Could you check a few things on this model? Use its own coordinates, in mm. A direction names the side the tool comes from. Round coordinates to 2 decimals unless told otherwise and drop trailing zeros. Loops run counter-clockwise (first coordinate to the right, second up) from the corner with the lowest first, then second, coordinate; pieces in that order, holes last.
from build123d import *

# Parameters (mm, degrees)
BOSS_EXTRUDE1_DEPTH = 300
SKETCH2_R           = 42.5
SKETCH2_W           = 5
SKETCH2_H           = 83.856690982
CUT_EXTRUDE1_DEPTH  = 349.855848061
SKETCH3_R           = 2
CUT_EXTRUDE2_DEPTH  = 349.855848061


with BuildPart() as part:
    # Sketch1 → Boss-Extrude1 (new body)
    with BuildSketch(Plane(origin=(0, 0, 0), x_dir=(0, 0, -1), z_dir=(1, 0, 0))):
        with BuildLine():
            Line((0, 0), (73.417375121, 0))
            ThreePointArc((73.417375121, 0), (79.943684732, -0.427756931), (86.358327376, -1.703708686))
            Line((86.358327376, -1.703708686), (176.592582629, -25.88190451))
            Line((176.592582629, -25.88190451), (175.816125494, -28.779681989))
            Line((175.816125494, -28.779681989), (85.58187024, -4.601486164))
            ThreePointArc((85.58187024, -4.601486164), (79.552106155, -3.402091515), (73.417375121, -3))
            Line((73.417375121, -3), (0, -3))
            Line((0, -3), (0, 0))
        make_face()
    extrude(amount=BOSS_EXTRUDE1_DEPTH)

    # Sketch2 → Cut-Extrude1 (cut, through all)
    with BuildSketch(Plane(origin=(0, 20, -5.358983849), x_dir=(1, 0, 0), z_dir=(0, 0.9659258262890681, -0.25881904510252174))):
        with Locations((48, 152.274066103)):
            Circle(SKETCH2_R)
        with Locations((252, 152.274066103)):
            Circle(SKETCH2_R)
        with Locations((48, -29.084261273)):
            Circle(SKETCH2_R)
        with Locations((252, -29.084261273)):
            Circle(SKETCH2_R)
        with Locations((2.5, 41.928345491)):
            Rectangle(SKETCH2_W, SKETCH2_H)
        with Locations((297.5, 41.928345491)):
            Rectangle(SKETCH2_W, SKETCH2_H)
    extrude(amount=-CUT_EXTRUDE1_DEPTH, mode=Mode.SUBTRACT)

    # Sketch3 → Cut-Extrude2 (cut, through all)
    with BuildSketch(Plane(origin=(0, 20, -5.358983849), x_dir=(1, 0, 0), z_dir=(0, 0.9659258262890681, -0.25881904510252174))):
        with Locations(Location((8, 87.856690982, 0), (0, 0, 270))):
            Circle(SKETCH3_R)
        with Locations(Location((8, 111.856690982, 0), (0, 0, 270))):
            Circle(SKETCH3_R)
        with Locations(Location((292, 87.856690982, 0), (0, 0, 270))):
            Circle(SKETCH3_R)
        with Locations(Location((292, 111.856690982, 0), (0, 0, 270))):
            Circle(SKETCH3_R)
    extrude(amount=-CUT_EXTRUDE2_DEPTH, mode=Mode.SUBTRACT)


solid = part.part
Item 1: Will these pins go through, and if not, where does the flat tip stop? pin 1 (22 mm diameter, centred on x = 118, z = -29, fed in from -Y); pin 2 (8 mm diameter, centred on x = 121, z = -80, fed in from +Y); pin 3 (8 mm diameter, centred on x = 147, z = -98.5, fed in from -Y).
Results list:
pin 1: stops at y = -3
pin 2: stops at y = -0.07
pin 3: stops at y = -9.13
Item 2: If we section it at B-B, the plane x = 213: Please give me the cut outline in (y, z).
Results list:
outline: (-28.78, -175.82) - (-25.88, -176.59) - (-23.78, -168.76) - (-26.68, -167.98) - close; (-17.94, -135.35) - (-15.04, -136.13) - (-1.7, -86.36) arc R50 ccw to (0, -73.42) - (0, 0) - (-3, 0) - (-3, -73.42) arc R47 cw to (-4.6, -85.58) - close
Item 3: If we section it at A-A, the plane x = 102: Please give me the cut outline in (y, z), then the cut area to 3 significant figures.
Results list:
outline: (-28.78, -175.82) - (-25.88, -176.59) - (-1.7, -86.36) arc R50 ccw to (0, -73.42) - (0, 0) - (-3, 0) - (-3, -73.42) arc R47 cw to (-4.6, -85.58) - close
area: 539 mm2
Item 4: If we section it at C-C, the plane z = -44: Please give me the cut outline in (x, y), then the cut area to 3 significant figures.
Results list:
outline: (5, -3) - (295, -3) - (295, 0) - (5, 0) - close
area: 870 mm2
Item 5: If I drill on line 1 along Y through (x, z) = (36, -16); line 2 along Y through (x, z) = (189.5, -154), over which ranges is the centre line in solid material (lowest first)?
Results list:
line 1: y = -3 to 0
line 2: y = -22.93 to -19.83
Item 6: We'd pull the mould along X, two halves only. Please class faces 3 (the cylindrical face through (147.97, -0.416, -79.853)), 4 (the flat face through (0, -15, -131)), 5 (the cylindrical face through (48.49, -2.82, -13.13)): released by +X, released by -X, zero draft, split by the parting line, or undercut.
Results list:
face 3: zero draft
face 4: released by -X
face 5: undercut
Item 7: If we section it at D-D, the plane y = -19.5: Count the separate pieces of the cut face and the enclosed holes in it, then the cut area to 3 significant figures.
Results list:
separate pieces: 3
enclosed holes: 0
area: 1,530 mm2
Item 8: For faces 1 (the flat face through (148, -3, -37)), 2 (the cylindrical face through (252.49, -2.82, -13.13)), which set-ups out of +Z, -Z, +X, -X, +Y, -Y let a thin tool reach every point of the face, with its end or its side?
Results list:
face 1: +Z, +X, -X, -Y
face 2: +Z, +Y
